Can you work these out from the model? Positions are in its coordinate system, mm. A direction names the side the tool comes from. Round coordinates to 2 decimals unless told otherwise and drop trailing zeros. Write each loop counter-clockwise with the first axis right and the second up, starting at its lowest first coordinate (ties: lowest second). Pieces come first, ordered by that corner, then holes.
Q1. I'm going to push a flat-ended pin straight in: pin 1 Ø1.5 at (y, z) = (-1.5, 19) entering from +X. Where does the tip first touch, or does it pass through?
Q2. If we section it at B-B (x = 0): Please give me the cut outline in (y, z) (3 decimals), plus the area to 3 significant figures.
Q3. If we section it at C-C (x = 45): Please give me the cut outline in (y, z).
Q4. Please list where these lines run through material, in increasing order: line 1 along X through (y, z) = (-2.75, -41); line 2 along Z through (x, y) = (32, -5.75); line 3 along X through (y, z) = (-5, 15).
Q5. If we section it at A-A (z = 0): Please give me the cut outline in (x, y) (3 decimals).
Q6. For faces 1 (the flat face through (13.417, -3.131, 82.28)), 2 (the flat face through (-2, 0, -91)), which set-ups out of +Z, -Z, +X, -X, +Y, -Y let a thin tool reach every point of the face, with its end or its side?
Q7. We'd pull the mould along Z, two halves only. Please class faces 3 (the flat face through (-2, -6.35, -91)), 4 (the cylindrical face through (-92.074, -3.131, -0.38)): +Z half, -Z half, draft (parallel to the pull), parting line (faces both ways), or undercut.
Q8. If we section it at D-D (z = 82.55): Please give me the cut outline in (x, y), plus the area to 3 significant figures.
from build123d import *

# Parameters (mm, degrees)
F0_R     = 139.7
F0_R_2   = 3.96875
F1_DEPTH = 6.35


with BuildPart() as f1:
    # F0 (on Front) → F1 (new body)
    with BuildSketch(Plane.XZ):
        Circle(F0_R)
        with Locations((-71.490397, -41.275)):
            Circle(F0_R_2, mode=Mode.SUBTRACT)
        with Locations((0, -82.55)):
            Circle(F0_R_2, mode=Mode.SUBTRACT)
        with Locations((71.490397, -41.275)):
            Circle(F0_R_2, mode=Mode.SUBTRACT)
        with Locations((-71.490397, 41.275)):
            Circle(F0_R_2, mode=Mode.SUBTRACT)
        with BuildLine():
            ThreePointArc((-67.231483, 62.910519), (-46.0375, 79.739289), (-20.866366, 89.679431))
            ThreePointArc((-20.866366, 89.679431), (-17.294985, 89.198071), (-14.94148, 86.469063))
            Line((-14.94148, 86.469063), (-11.934096, 78.206344))
            ThreePointArc((-11.934096, 78.206344), (-10.300747, 75.121366), (-7.889211, 72.597596))
            ThreePointArc((-7.889211, 72.597596), (0, 73.025), (7.889211, 72.597596))
            ThreePointArc((7.889211, 72.597596), (10.300747, 75.121366), (11.934096, 78.206344))
            Line((11.934096, 78.206344), (14.94148, 86.469063))
            ThreePointArc((14.94148, 86.469063), (17.294985, 89.198071), (20.866366, 89.679431))
            ThreePointArc((20.866366, 89.679431), (46.0375, 79.739289), (67.231483, 62.910519))
            ThreePointArc((67.231483, 62.910519), (68.600303, 59.576932), (67.413665, 56.174233))
            Line((67.413665, 56.174233), (61.761633, 49.438403))
            ThreePointArc((61.761633, 49.438403), (59.906638, 46.481392), (58.926757, 43.131056))
            ThreePointArc((58.926757, 43.131056), (63.241505, 36.5125), (66.815968, 29.466541))
            ThreePointArc((66.815968, 29.466541), (70.207385, 28.639974), (73.695729, 28.767942))
            Line((73.695729, 28.767942), (82.355145, 30.29483))
            ThreePointArc((82.355145, 30.29483), (85.895288, 29.621139), (88.097849, 26.768912))
            ThreePointArc((88.097849, 26.768912), (92.075, 0), (88.097849, -26.768912))
            ThreePointArc((88.097849, -26.768912), (85.895288, -29.621139), (82.355145, -30.29483))
            Line((82.355145, -30.29483), (73.695729, -28.767942))
            ThreePointArc((73.695729, -28.767942), (70.207385, -28.639974), (66.815968, -29.466541))
            ThreePointArc((66.815968, -29.466541), (63.241505, -36.5125), (58.926757, -43.131056))
            ThreePointArc((58.926757, -43.131056), (59.906638, -46.481392), (61.761633, -49.438403))
            Line((61.761633, -49.438403), (67.413665, -56.174233))
            ThreePointArc((67.413665, -56.174233), (68.600303, -59.576932), (67.231483, -62.910519))
            ThreePointArc((67.231483, -62.910519), (46.0375, -79.739289), (20.866366, -89.679431))
            ThreePointArc((20.866366, -89.679431), (17.294985, -89.198071), (14.94148, -86.469063))
            Line((14.94148, -86.469063), (11.934096, -78.206344))
            ThreePointArc((11.934096, -78.206344), (10.300747, -75.121366), (7.889211, -72.597596))
            ThreePointArc((7.889211, -72.597596), (0, -73.025), (-7.889211, -72.597596))
            ThreePointArc((-7.889211, -72.597596), (-10.300747, -75.121366), (-11.934096, -78.206344))
            Line((-11.934096, -78.206344), (-14.94148, -86.469063))
            ThreePointArc((-14.94148, -86.469063), (-17.294985, -89.198071), (-20.866366, -89.679431))
            ThreePointArc((-20.866366, -89.679431), (-46.0375, -79.739289), (-67.231483, -62.910519))
            ThreePointArc((-67.231483, -62.910519), (-68.600303, -59.576932), (-67.413665, -56.174233))
            Line((-67.413665, -56.174233), (-61.761633, -49.438403))
            ThreePointArc((-61.761633, -49.438403), (-59.906638, -46.481392), (-58.926757, -43.131056))
            ThreePointArc((-58.926757, -43.131056), (-63.241505, -36.5125), (-66.815968, -29.466541))
            ThreePointArc((-66.815968, -29.466541), (-70.207385, -28.639974), (-73.695729, -28.767942))
            Line((-73.695729, -28.767942), (-82.355145, -30.29483))
            ThreePointArc((-82.355145, -30.29483), (-85.895288, -29.621139), (-88.097849, -26.768912))
            ThreePointArc((-88.097849, -26.768912), (-92.075, 0), (-88.097849, 26.768912))
            ThreePointArc((-88.097849, 26.768912), (-85.895288, 29.621139), (-82.355145, 30.29483))
            Line((-82.355145, 30.29483), (-73.695729, 28.767942))
            ThreePointArc((-73.695729, 28.767942), (-70.207385, 28.639974), (-66.815968, 29.466541))
            ThreePointArc((-66.815968, 29.466541), (-63.241505, 36.5125), (-58.926757, 43.131056))
            ThreePointArc((-58.926757, 43.131056), (-59.906638, 46.481392), (-61.761633, 49.438403))
            Line((-61.761633, 49.438403), (-67.413665, 56.174233))
            ThreePointArc((-67.413665, 56.174233), (-68.600303, 59.576932), (-67.231483, 62.910519))
        make_face(mode=Mode.SUBTRACT)
        with Locations((71.490397, 41.275)):
            Circle(F0_R_2, mode=Mode.SUBTRACT)
        with Locations((0, 82.55)):
            Circle(F0_R_2, mode=Mode.SUBTRACT)
    extrude(amount=F1_DEPTH)


solid = f1.part
A:
1. pin 1: stops at x = 138.5
2. outline: (-6.35, -139.7) - (0, -139.7) - (0, -86.519) - (-6.35, -86.519) - close; (-6.35, -78.581) - (0, -78.581) - (0, -73.025) - (-6.35, -73.025) - close; (-6.35, 73.025) - (0, 73.025) - (0, 78.581) - (-6.35, 78.581) - close; (-6.35, 86.519) - (0, 86.519) - (0, 139.7) - (-6.35, 139.7) - close
2. area: 746 mm2
3. outline: (-6.35, -132.25) - (0, -132.25) - (0, -80.33) - (-6.35, -80.33) - close; (-6.35, 80.33) - (0, 80.33) - (0, 132.25) - (-6.35, 132.25) - close
4. line 1: x = -133.55 to -75.45, -67.53 to -60.43, 60.43 to 67.53, 75.45 to 133.55
4. line 2: z = -135.99 to -86.34, 86.34 to 135.99
4. line 3: x = -138.89 to -90.84, 90.84 to 138.89
5. outline: (-139.7, -6.35) - (-92.075, -6.35) - (-92.075, 0) - (-139.7, 0) - close; (92.075, -6.35) - (139.7, -6.35) - (139.7, 0) - (92.075, 0) - close
6. face 1: +Y, -Y
6. face 2: +Z, -Z, +X, -X, +Y
7. face 3: draft
7. face 4: undercut
8. outline: (-112.7, -6.35) - (-40.78, -6.35) - (-40.78, 0) - (-112.7, 0) - close; (-13.52, -6.35) - (-3.97, -6.35) - (-3.97, 0) - (-13.52, 0) - close; (3.97, -6.35) - (13.52, -6.35) - (13.52, 0) - (3.97, 0) - close; (40.78, -6.35) - (112.7, -6.35) - (112.7, 0) - (40.78, 0) - close
8. area: 1,030 mm2
